Autodesk Inventor part; units mm, degrees
ref_plane "YZ Plane" through (0, 0, 0) normal (1, 0, 0) x (0, 1, 0)
ref_plane "XZ Plane" through (0, 0, 0) normal (0, 1, 0) x (-1, 0, 0)
ref_plane "XY Plane" through (0, 0, 0) normal (0, 0, 1) x (1, 0, 0)
sketch "Boceto1" plane through (0, 0, 0) normal (0, 0, 1) x (1, 0, 0)
  line L0 (-2.4, 3.4) -> (2.4, 3.4)
  line L1 (2.4, 3.4) -> (2.4, -3.4)
  line L2 (2.4, -3.4) -> (-2.4, -3.4)
  line L3 (-2.4, -3.4) -> (-2.4, 3.4)
  line L4 (0, -4.76) -> (0, 4.76)
  line L5 (-3.36, 0) -> (3.36, 0)
  line L6 (-1.4, 2.2) -> (0.5, 2.2)
  line L7 (0.5, 2.2) -> (0.5, -2.2)
  line L8 (0.5, -2.2) -> (-1.4, -2.2)
  line L9 (-1.4, -2.2) -> (-1.4, 2.2)
  dimension "d0" = 4.8
  dimension "d1" = 6.8
  dimension "d19" = 1.9
  dimension "d20" = 4.4
  dimension "d21" = 1
extrude "Extrusión1" add sketch "Boceto1" along normal blind 7 contours L0 L4 L6 L9 L5 L3 | L0 L1 L5 L7 L6 L4 | L5 L9 L8 L4 L2 L3 | L1 L2 L4 L8 L7 L5
sketch "Boceto2" plane through (2.4, -3.4, 0) normal (1, 0, 0) x (0, 0, -1)
  line L0 (-1.2, 4.8904) -> (-2.2, 4.8904)
  line L1 (-2.2, 4.8904) -> (-2.2, 1.9096)
  line L2 (-2.2, 1.9096) -> (-1.2, 1.9096)
  line L3 (-1.2, 1.9096) -> (-1.2, 4.8904)
  line L4 (1.4, 3.4) -> (-8.4, 3.4)
  line L5 (0, 0) -> (0, 6.8)
  point P0 (0, 3.4)
  dimension "d8" = 1.2
  dimension "d9" = 1
extrude "Extrusión2" add sketch "Boceto2" along normal blind 0.3
sketch "Boceto3" plane through (-2.4, 3.4, 0) normal (0, 1, 0) x (1, 0, 0)
  line L0 (4.8, 0) -> (0, 0)
  line L1 (4.8, 0) -> (4.8, -0.8)
  line L2 (4.8, 0) -> (4.8, -7)
  line L3 (4.8, -0.8) -> (5.3, 0)
  line L4 (5.3, 0) -> (4.8, 0)
  point P0 (2.4, 0)
  dimension "d12" = 0.8
  dimension "d22" = 0.5
extrude "Extrusión3" add sketch "Boceto3" against normal blind 1
fillet "Empalme1" radius 0.3 1 edges at (2.7, 0, 2.2)
mirror "Simetría1" about plane through (0, 0, 0) normal (1, 0, 0) of "Extrusión2", "Empalme1"
mirror "Simetría2" about plane through (0, 0, 0) normal (1, 0, 0) of "Extrusión3"
mirror "Simetría3" about plane through (0, 0, 0) normal (0, 1, 0) of "Extrusión3", "Simetría2"
sketch "Boceto4" plane through (0, 0, 0) normal (0, 0, -1) x (-1, 0, 0)
  line L0 (-2.9, 3.4) -> (2.9, 3.4)
  line L1 (-2.9, 3.4) -> (-2.9, 2.4)
  line L2 (-2.4, 2.4) -> (-2.9, 2.4)
  line L3 (-2.4, -2.4) -> (-2.4, 2.4)
  line L4 (-2.4, -2.4) -> (-2.9, -2.4)
  line L5 (-2.9, -3.4) -> (-2.9, -2.4)
  line L6 (2.9, -3.4) -> (-2.9, -3.4)
  line L7 (2.9, -3.4) -> (2.9, -2.4)
  line L8 (2.4, -2.4) -> (2.9, -2.4)
  line L9 (2.4, 2.4) -> (2.4, -2.4)
  line L10 (2.4, 2.4) -> (2.9, 2.4)
  line L11 (2.9, 3.4) -> (2.9, 2.4)
  line L12 (2.4, -3.4) -> (-2.4, -3.4)
  line L13 (-2.4, -3.4) -> (-2.4, 3.4)
  line L14 (2.4, -3.4) -> (-2.4, -3.4)
  line L15 (-2.4, -3.4) -> (-2.4, 3.4)
  line L16 (-2.4, 3.4) -> (2.4, 3.4)
  line L17 (2.4, 3.4) -> (2.4, -3.4)
  point P0 (0, 0)
extrude "Extrusión4" add sketch "Boceto4" against normal blind 0.6 contours L0 L17 L9 L6 L13 L3
properties part number "Porta Hall Sensor"
The model under review builds one solid part; all positions refer to its coordinate system, in mm. A direction names the side the tool comes from. Give positions to 0.01 mm unless a question says otherwise; leave off trailing zeros. Write each loop counter-clockwise with the first axis right and the second up, starting at its lowest first coordinate (ties: lowest second). Pieces come first, ordered by that corner, then holes. Notation, with made-up numbers: M -20,43.25 L 24,43.25 A10 cw 24,58.25 Z; hole C 80,-31.5 d3. An arc over 180 degrees is marked long. Write each question's results on one line, items separated by ' | '. Start each with the question number.
1. Insertion check: pin 1 Ø0.6 at (y, z) = (-0.5, 1.5) entering from -X; pin 2 Ø2 at (y, z) = (0, 4) entering from -X; pin 3 Ø2 at (y, z) = (0, 5) entering from +X. Each pin has a flat end and moves straight along its axis. Give the tip position at first contact, or say it passes through.
2. We need section D-D (y = 2). Write out the cut boundary in (x, z), and give its area (3 significant figures).
3. For probe 1 along X at (y, z) = (2, 2.25); probe 2 along Y at (x, z) = (-0.4, 4.25); probe 3 along X at (y, z) = (3, 3.25), list the stretches that pass through material, from the lowest coordinate up. Write a range as [from, to].
4. We need section C-C (x = -1.05). Write out the cut boundary in (y, z), and give its area (3 significant figures).
5. For faces 1 (the flat face through (0, 0, 0)), 2 (the flat face through (0.5, 0, 4)), list the 3-axis set-ups (+Z, -Z, +X, -X, +Y, -Y) from which the entire face can be reached by the end or side of a thin tool; tool diameter is ignored.
6. We need section B-B (z = 5). Write out the cut boundary in (x, y).
7. Mouldability with a two-part tool opening along X and no side actions: class faces 3 (the flat face through (0, -2.2, 4)), 4 (the flat face through (-1.4, 0, 4)), 5 (the flat face through (1, 0, 7)) as released by +X, released by -X, zero draft, split by the parting line, or undercut.
Results found:
1) pin 1: stops at x = -2.7 | pin 2: stops at x = -2.4 | pin 3: stops at x = 2.4
2) outline: M -2.4,0 L 2.4,0 L 2.4,7 L 0.5,7 L 0.5,0.6 L -1.4,0.6 L -1.4,7 L -2.4,7 Z | area: 21.4 mm^2
3) probe 1: x = [-2.4, -1.4], [0.5, 2.4] | probe 2: y = [-3.4, -2.2], [2.2, 3.4] | probe 3: x = [-2.4, 2.4]
4) outline: M -3.4,0 L 3.4,0 L 3.4,7 L 2.2,7 L 2.2,0.6 L -2.2,0.6 L -2.2,7 L -3.4,7 Z | area: 19.4 mm^2
5) face 1: -Z, +X, -X, +Y, -Y | face 2: +Z
6) outline: M -2.4,-3.4 L 2.4,-3.4 L 2.4,3.4 L -2.4,3.4 Z; hole M -1.4,-2.2 L 0.5,-2.2 L 0.5,2.2 L -1.4,2.2 Z
7) face 3: undercut | face 4: undercut | face 5: zero draft
